Here's how the part is built. I have some questions about the finished solid (model axes, mm). Round coordinates to 2 decimals unless told otherwise and drop trailing zeros. Order: outer loops, then holes, each group sorted by start corner. A loop starts at its lowest first (then second) coordinate and runs counter-clockwise, first axis right, second up. Notation, with made-up numbers: (50.5, 68) - (73.5, 68) arc R22 cw to (73.5, 102) - close; hole circle Ø3 at (0, -36.5). An arc over 180 degrees is marked (long way). Answer as a JSON object with one key per item and string values.
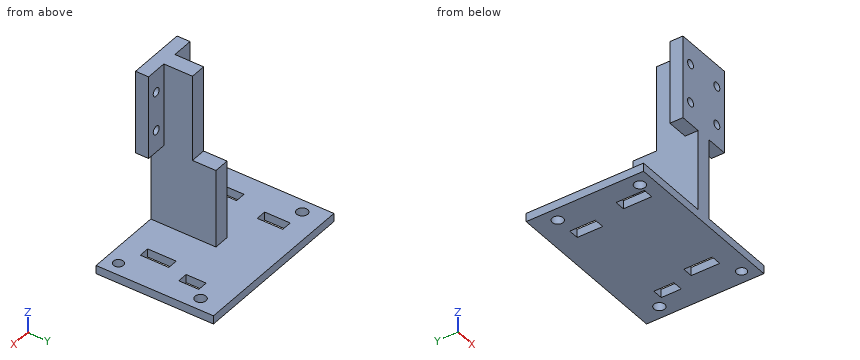
```python
from build123d import *

# Parameters (mm, degrees)
SKETCH_1_W          = 8.2
SKETCH_1_H          = 32
SKETCH_1_R          = 1.6
EXTRUDE_1_DEPTH     = 5
SKETCH_2_W          = 6
SKETCH_2_H          = 63
EXTRUDE_2_DEPTH     = 25
SKETCH_3_W          = 65
SKETCH_3_H          = 45
EXTRUDE_3_DEPTH     = 3.2
SKETCH_4_R          = 1.922469011
SKETCH_4_R_2        = 2.1
CUT_EXTRUDE_1_DEPTH = 13.2
SKETCH_7_W          = 4
SKETCH_7_H          = 7.68275579
SKETCH_7_H_2        = 10.940540448
SKETCH_7_H_3        = 9.798767364
SKETCH_7_H_4        = 10.843668011
CUT_EXTRUDE_2_DEPTH = 13.2
SKETCH_8_W          = 33
SKETCH_8_H          = 9
CUT_EXTRUDE_3_DEPTH = 13.2


with BuildPart() as part:
    # 草图1 → 凸台-拉伸1 (new body)
    with BuildSketch(Plane(origin=(0, 0, 0), x_dir=(1, 0, 0), z_dir=(0, 1, 0))):
        Rectangle(SKETCH_1_W, SKETCH_1_H)
        with Locations(Location((0, 7.5, 0), (0, 0, 270))):
            Circle(SKETCH_1_R, mode=Mode.SUBTRACT)
        with Locations(Location((0, -7.5, 0), (0, 0, 90))):
            Circle(SKETCH_1_R, mode=Mode.SUBTRACT)
    extrude_1 = extrude(amount=EXTRUDE_1_DEPTH)

    # 草图2 → 凸台-拉伸2 (add)
    with BuildSketch(Plane(origin=(0, 0, 0), x_dir=(1, 0, 0), z_dir=(0, 1, 0))):
        with Locations((7.1, 15.5)):
            Rectangle(SKETCH_2_W, SKETCH_2_H)
    extrude(amount=EXTRUDE_2_DEPTH)

    # 草图3 → 凸台-拉伸3 (add)
    with BuildSketch(Plane(origin=(0, 0, -47), x_dir=(-1, 0, 0), z_dir=(0, 0, -1))):
        with Locations((-7.1, 22.5)):
            Rectangle(SKETCH_3_W, SKETCH_3_H)
    extrude(amount=EXTRUDE_3_DEPTH)

    # 草图4 → 切除-拉伸1 (cut)
    with BuildSketch(Plane(origin=(0, 0, -50.2), x_dir=(-1, 0, 0), z_dir=(0, 0, -1))):
        with Locations((-34.6, 5)):
            Circle(SKETCH_4_R)
        with Locations((20.3, 5)):
            Circle(SKETCH_4_R_2)
        with Locations((-34.6, 36.5)):
            Circle(SKETCH_4_R_2)
        with Locations((20.3, 36.5)):
            Circle(SKETCH_4_R_2)
    extrude(amount=-CUT_EXTRUDE_1_DEPTH, mode=Mode.SUBTRACT)

    # 草图7 → 切除-拉伸2 (cut)
    with BuildSketch(Plane(origin=(0, 0, -50.2), x_dir=(-1, 0, 0), z_dir=(0, 0, -1))):
        with Locations((-29.100303776, 29.48244197)):
            Rectangle(SKETCH_7_W, SKETCH_7_H)
        with Locations((-25.252299823, 13.640004416)):
            Rectangle(SKETCH_7_W, SKETCH_7_H_2)
        with Locations((11.465466314, 31.834080816)):
            Rectangle(SKETCH_7_W, SKETCH_7_H_3)
        with Locations((15.188894487, 10.930624409)):
            Rectangle(SKETCH_7_W, SKETCH_7_H_4)
    extrude(amount=-CUT_EXTRUDE_2_DEPTH, mode=Mode.SUBTRACT)

    # 镜向1: 凸台-拉伸1 across plane
    add(extrude_1.mirror(Plane.ZY.offset(-7.1)))

    # 草图8 → 切除-拉伸3 (cut)
    with BuildSketch(Plane.ZY.offset(-4.1)):
        with Locations((-0.5, 20.5)):
            Rectangle(SKETCH_8_W, SKETCH_8_H)
    extrude(amount=-CUT_EXTRUDE_3_DEPTH, mode=Mode.SUBTRACT)


solid = part.part
```
1. Imagine slicing it at D-D (x = 34.6). List the corners of the cut face in (y, z) for me, plus the area to 3 significant figures.
Responses:
{"outline": "(0, -50.2) - (3.08, -50.2) - (3.08, -47) - (0, -47) - close; (6.92, -50.2) - (34.4, -50.2) - (34.4, -47) - (6.92, -47) - close; (38.6, -50.2) - (45, -50.2) - (45, -47) - (38.6, -47) - close", "area": "118 mm2"}
2. Imagine slicing it at C-C (y = 28). List the corners of the cut face in (x, z) for me, plus the area to 3 significant figures.
Responses:
{"outline": "(-25.4, -50.2) - (-13.47, -50.2) - (-13.47, -47) - (-25.4, -47) - close; (-9.47, -50.2) - (27.1, -50.2) - (27.1, -47) - (-9.47, -47) - close; (31.1, -50.2) - (39.6, -50.2) - (39.6, -47) - (31.1, -47) - close", "area": "182 mm2"}
3. If I drill on L1, parallel to Y at x = 34.6, z = -48.9; L2, parallel to Y at x = -20.3, z = -48.5; L3, parallel to Z at x = 10.5, y = 17, over which ranges is the centre line in solid material (lowest first)? Write a range as [from, to].
Responses:
{"L1": "[0, 3.08], [6.92, 34.4], [38.6, 45]", "L2": "[0, 2.9], [7.1, 34.4], [38.6, 45]", "L3": "[-50.2, -47]"}
4. Imagine slicing it at A-A (z = -7.5). List the corners of the cut face in (x, y) for me.
Responses:
{"outline": "(-4.1, 0) - (-1.6, 0) - (-1.6, 5) - (-4.1, 5) - close; (1.6, 0) - (12.6, 0) - (12.6, 5) - (10.1, 5) - (10.1, 16) - (4.1, 16) - (4.1, 5) - (1.6, 5) - close; (15.8, 0) - (18.3, 0) - (18.3, 5) - (15.8, 5) - close"}
5. Imagine slicing it at B-B (x = 14.2). List the corners of the cut face in (y, z) for me, plus the area to 3 significant figures.
Responses:
{"outline": "(0, -50.2) - (45, -50.2) - (45, -47) - (0, -47) - close; (0, -16) - (5, -16) - (5, -9.1) - (0, -9.1) - close; (0, -5.9) - (5, -5.9) - (5, 5.9) - (0, 5.9) - close; (0, 9.1) - (5, 9.1) - (5, 16) - (0, 16) - close", "area": "272 mm2"}
6. For P1, Ø12.5, axis at y = 11.5, z = -6, coming from the -X side; P2, Ø9, axis at x = 14, z = 3.5, coming from the +Y side; P3, Ø4, axis at x = 14.2, z = 7.5, coming from the +Y side, each with a flat end and sliding along its axis, tell me the tip position at first contact or that it passes through.
Responses:
{"P1": "x = 4.1", "P2": "y = 16", "P3": "y = 5"}
